Autodesk Inventor part; units mm, degrees
ref_plane "YZ Plane" through (0, 0, 0) normal (1, 0, 0) x (0, 1, 0)
ref_plane "XZ Plane" through (0, 0, 0) normal (0, 1, 0) x (-1, 0, 0)
ref_plane "XY Plane" through (0, 0, 0) normal (0, 0, 1) x (1, 0, 0)
sketch "Sketch1" plane through (0, 0, 0) normal (0, 0, 1) x (1, 0, 0)
  point P0 (0, 0)
sketch "Sketch2" plane through (0, 0, 0) normal (0, 0, 1) x (1, 0, 0)
  circle A0 centre (0, 0) radius 22.5
  dimension "d0" = 45
extrude "Extrusion1" add sketch "Sketch2" along normal blind 10
sketch "Sketch3" plane through (0, 0, 10) normal (0, 0, 1) x (1, 0, 0)
  line L0 (-3.75, 15) -> (3.75, 15)
  line L1 (3.75, 15) -> (3.75, -28)
  line L2 (3.75, -28) -> (-3.75, -28)
  line L3 (-3.75, -28) -> (-3.75, 15)
  point P0 (0, 0)
  dimension "d3" = 7.5
  dimension "d4" = 43
  dimension "d6" = 3.75
  dimension "d7" = 15
extrude "Extrusion2" cut sketch "Sketch3" against normal blind 10
sketch "Sketch4" plane through (0, 0, 10) normal (0, 0, 1) x (1, 0, 0)
  circle A0 centre (0, 0) radius 7.5
  dimension "d10" = 15
extrude "Extrusion3" cut sketch "Sketch4" against normal blind 10
properties part number "plate"
Here's how the part is built. I have some questions about the finished solid (model axes, mm). A direction names the side the tool comes from. Coordinates: 2 decimals unless noted, no trailing zeros. Order: outer loops, then holes, each group sorted by start corner. A loop starts at its lowest first (then second) coordinate and runs counter-clockwise, first axis right, second up. Notation, with made-up numbers: (76, 79) - (120, 79) arc R8 cw to (120, 85) - close; hole circle Ø6 at (-34, 81.5). An arc over 180 degrees is marked (long way). One line per question, with ' | ' between items.
(1) Suppose I cut it at B-B on z = 7. List the corners of the cut face in (x, y) for me, and give its area (3 significant figures).
Report:
outline: (-3.75, -22.19) - (-3.75, -6.5) arc R7.5 cw to (-3.75, 6.5) - (-3.75, 15) - (3.75, 15) - (3.75, 6.5) arc R7.5 cw to (3.75, -6.5) - (3.75, -22.19) arc R22.5 ccw (long way) to start | area: 1,240 mm2
(2) If I drill on L1, parallel to X at y = -7, z = 6.75; L2, parallel to X at y = 2, z = 4.5; L3, parallel to Y at x = 0, z = 1, over which ranges is the centre line in solid material (lowest first)?
Report:
L1: x = -21.38 to -3.75, 3.75 to 21.38 | L2: x = -22.41 to -7.23, 7.23 to 22.41 | L3: y = 15 to 22.5
(3) Suppose I cut it at C-C on x = 0. List the corners of the cut face in (y, z) for me.
Report:
outline: (15, 0) - (22.5, 0) - (22.5, 10) - (15, 10) - close
(4) Suppose I cut it at D-D on y = 5. List the corners of the cut face in (x, z) for me, and give its area (3 significant figures).
Report:
outline: (-21.94, 0) - (-5.59, 0) - (-5.59, 10) - (-21.94, 10) - close; (5.59, 0) - (21.94, 0) - (21.94, 10) - (5.59, 10) - close | area: 327 mm2
(5) For faces 4 (the flat face through (3.75, 11, 5)), 5 (the flat face through (10, 0, 0)), 6 (the cylindrical face through (7.5, -0.1, 5.1)), which set-ups out of +Z, -Z, +X, -X, +Y, -Y let a thin tool reach every point of the face, with its end or its side?
Report:
face 4: +Z, -Z, -Y | face 5: -Z, +X, -X, +Y, -Y | face 6: +Z, -Z
(6) Suppose I cut it at A-A on y = 0. List the corners of the cut face in (x, z) for me.
Report:
outline: (-22.5, 0) - (-7.5, 0) - (-7.5, 10) - (-22.5, 10) - close; (7.5, 0) - (22.5, 0) - (22.5, 10) - (7.5, 10) - close
(7) Will these pins go through, and if not, where does the flat tip stop? pin 1 (1 mm diameter, centred on x = 1, z = 2, fed in from +Y); pin 2 (2 mm diameter, centred on x = -15.5, z = 6, fed in from +Y); pin 3 (4.5 mm diameter, centred on y = 9, z = 3, fed in from -X); pin 4 (3 mm diameter, centred on x = 4.5, z = 7.5, fed in from -Y).
Report:
pin 1: stops at y = 22.49 | pin 2: stops at y = 17.2 | pin 3: stops at x = -21.46 | pin 4: stops at y = -22.19
(8) If we mould it in two halves opening along X, with no side actions, what happens to faces 1 (the cylindrical face through (-7.5, 0.1, 5.1)), 2 (the cylindrical face through (-0.94, 22.48, 4.93)), 3 (the flat face through (10, 0, 10))? For each: pulls with the +X half, pulls with the -X half, needs draft (parallel to the pull), parting line crosses it, or undercut.
Report:
face 1: undercut | face 2: parting line crosses it | face 3: needs draft
